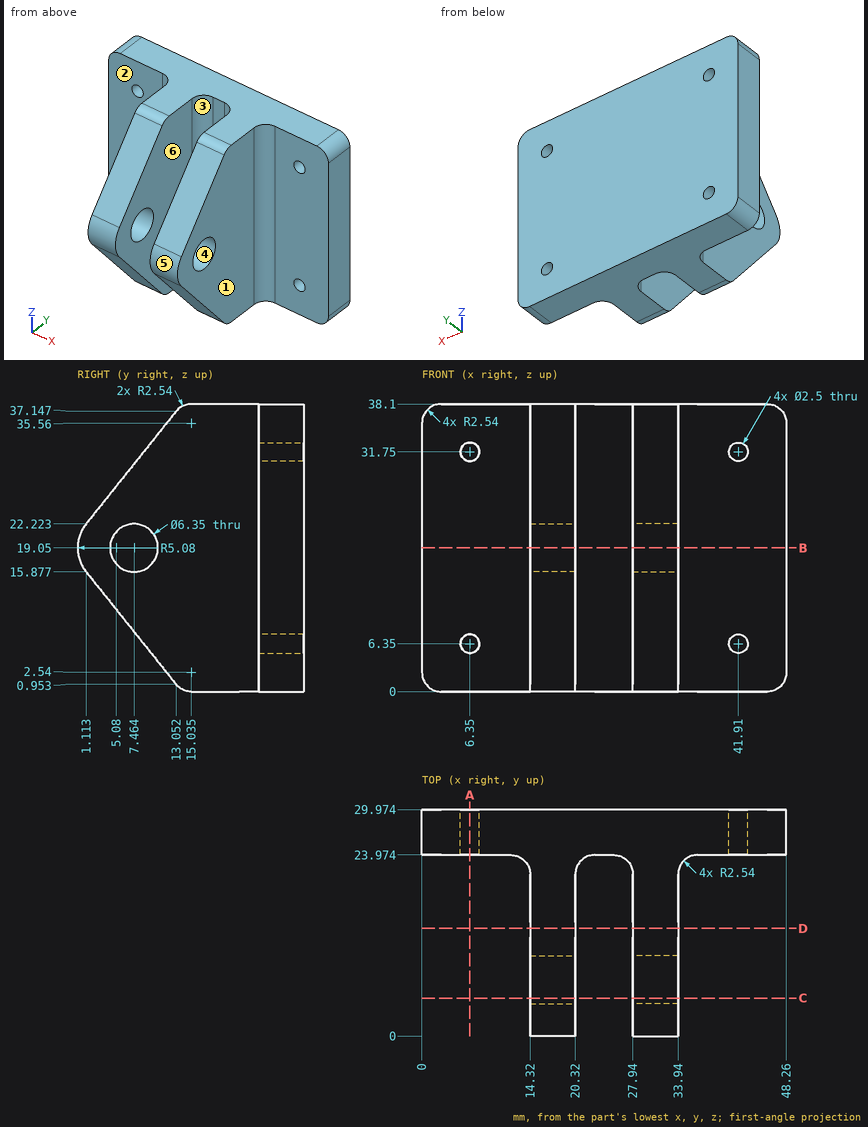
For this review, use the dimensioned drawing (mm, ordinates from the lowest corner) and the shaded views. A direction names the side the tool comes from. Coordinates: 2 decimals unless noted, no trailing zeros. Loops run counter-clockwise (first coordinate to the right, second up) from the corner with the lowest first, then second, coordinate; pieces in that order, holes last. Notation, with made-up numbers: (-25.5, 41.25) -> (33.5, 41.25) arc R17 ccw to (33.5, 71.25) -> close; hole circle Ø10 at (-4, -26). An arc over 180 degrees is marked (long way). Write each question's results on one line, items separated by ' | '.
Q1. Add section D-D, the plane y = 14.25. State the section outline as (x, z) points (1 decimal), then the cut area to 3 significant figures.
Taken from the geometry:
outline: (14.3, 0.1) -> (20.3, 0.1) -> (20.3, 38) -> (14.3, 38) -> close; (27.9, 0.1) -> (33.9, 0.1) -> (33.9, 38) -> (27.9, 38) -> close | area: 454 mm²
Q2. To check wall thickness, follow line 1 along X through (y, z) = (28.55, 31.75); line 2 along Z through (x, y) = (6.35, 25.8); line 3 along X through (y, z) = (9.75, 26.5). State the ranges of each line that lie inside material, in increasing order. Write a range as [from, to].
Taken from the geometry:
line 1: [0, 5.1], [7.6, 40.66], [43.16, 48.26] | line 2: [0, 5.1], [7.6, 30.5], [33, 38.1] | line 3: [14.32, 20.32], [27.94, 33.94]
Q3. Machinability: for the marked faces 1, 2 and 3, which of the approach directions +Z, -Z, +X, -X, +Y, -Y give a long, thin tool a straight path to every point of the face, cutting with its end or side? Answer none if there is none.
Taken from the geometry:
face 1: +Z, -Z, +X, -Y | face 2: +Z, -Z, -X, -Y | face 3: +Z, -Z, -Y
Q4. Add section A-A, the plane x = 6.35. State the section outline as (y, z) points (1 decimal).
Taken from the geometry:
outline: (24, 0) -> (30, 0) -> (30, 5.1) -> (24, 5.1) -> close; (24, 7.6) -> (30, 7.6) -> (30, 30.5) -> (24, 30.5) -> close; (24, 33) -> (30, 33) -> (30, 38.1) -> (24, 38.1) -> close
Q5. Add section B-B, the plane z = 19.05. State the section outline as (x, y) points (1 decimal).
Taken from the geometry:
outline: (0, 24) -> (11.8, 24) arc R2.5 cw to (14.3, 21.4) -> (14.3, 10.6) -> (20.3, 10.6) -> (20.3, 21.4) arc R2.5 cw to (22.9, 24) -> (25.4, 24) arc R2.5 cw to (27.9, 21.4) -> (27.9, 10.6) -> (33.9, 10.6) -> (33.9, 21.4) arc R2.5 cw to (36.5, 24) -> (48.3, 24) -> (48.3, 30) -> (0, 30) -> close; (14.3, 0) -> (20.3, 0) -> (20.3, 4.3) -> (14.3, 4.3) -> close; (27.9, 0) -> (33.9, 0) -> (33.9, 4.3) -> (27.9, 4.3) -> close
Q6. Mouldability with a two-part tool opening along Z and no side actions: class the marked faces 4, 5 and 6 as +Z half, -Z half, draft (parallel to the pull), parting line (faces both ways), or undercut.
Taken from the geometry:
face 4: undercut | face 5: parting line | face 6: draft
Q7. For pin 1 Ø2 at (y, z) = (4, 13.5) entering from +X; pin 2 Ø1.5 at (x, z) = (6.35, 6.35) entering from +Y; pin 3 Ø0.8 at (x, z) = (24, 20.5) entering from -Y; pin 4 Ø17 at (y, z) = (11, 27.5) entering from -X, all flat-tipped, find the tip position at first contact; note any pin that passes through.
Taken from the geometry:
pin 1: x = 33.94 | pin 2: through | pin 3: y = 23.97 | pin 4: x = 14.32
Q8. Add section C-C, the plane y = 5. State the section outline as (x, z) points, then the cut area to 3 significant figures.
Taken from the geometry:
outline: (14.32, 11.02) -> (20.32, 11.02) -> (20.32, 17.05) -> (14.32, 17.05) -> close; (14.32, 21.05) -> (20.32, 21.05) -> (20.32, 27.08) -> (14.32, 27.08) -> close; (27.94, 11.02) -> (33.94, 11.02) -> (33.94, 17.05) -> (27.94, 17.05) -> close; (27.94, 21.05) -> (33.94, 21.05) -> (33.94, 27.08) -> (27.94, 27.08) -> close | area: 145 mm²
